```python
from build123d import *

# Parameters (mm, degrees)
BOSS_EXTRUDE1_DEPTH      = 4.9
BOSS_EXTRUDE1_DEPTH_BACK = 4.9


with BuildPart() as part:
    # Sketch1 → Boss-Extrude1 (new, two sides: drawn at the far end of the back side and taken through both)
    with BuildSketch(Plane(origin=(0, 0, 0), x_dir=(1, 0, 0), z_dir=(0, 1, 0)).offset(-BOSS_EXTRUDE1_DEPTH_BACK)):
        with BuildLine():
            Line((14.139704236, -107.57296828), (14.139704236, -55))
            Line((14.139704236, -55), (11.139704236, -55))
            Line((11.139704236, -55), (11.139704236, -107.57296828))
            ThreePointArc((11.139704236, -107.57296828), (11.954116062, -129.773650702), (14.392973543, -151.854989901))
            Line((14.392973543, -151.854989901), (34.78314741, -289.876871715))
            ThreePointArc((34.78314741, -289.876871715), (36.798345533, -293.542093696), (40.718726235, -295))
            Line((40.718726235, -295), (62.036020432, -295))
            ThreePointArc((62.036020432, -295), (63.863676368, -294.379006889), (64.934691141, -292.773115853))
            Line((64.934691141, -292.773115853), (69.645825561, -275.109492351))
            ThreePointArc((69.645825561, -275.109492351), (69.730627927, -274.02191122), (69.420940845, -272.975910231))
            Line((69.420940845, -272.975910231), (67.998466185, -270.180256335))
            Line((67.998466185, -270.180256335), (67.934740393, -270.07233274))
            Line((67.934740393, -270.07233274), (65.932760352, -266.681854911))
            ThreePointArc((65.932760352, -266.681854911), (65.317615772, -266.221021537), (64.557173026, -266.332811892))
            Line((64.557173026, -266.332811892), (63.276988126, -267.100922833))
            ThreePointArc((63.276988126, -267.100922833), (63.049164753, -267.408401483), (63.10548954, -267.786917173))
            Line((63.10548954, -267.786917173), (65.42072044, -271.645635339))
            Line((65.42072044, -271.645635339), (65.805438483, -272.286832078))
            ThreePointArc((65.805438483, -272.286832078), (65.89276832, -272.442724972), (65.970662013, -272.603540604))
            Line((65.970662013, -272.603540604), (66.311869933, -273.364986559))
            ThreePointArc((66.311869933, -273.364986559), (66.564497004, -274.351078344), (66.472838335, -275.364881152))
            Line((66.472838335, -275.364881152), (62.629961452, -289.773115853))
            ThreePointArc((62.629961452, -289.773115853), (61.558946679, -291.379006889), (59.731290743, -292))
            Line((59.731290743, -292), (43.308092042, -292))
            ThreePointArc((43.308092042, -292), (39.387711339, -290.542093696), (37.372513216, -286.876871715))
            Line((37.372513216, -286.876871715), (17.360762956, -151.416554044))
            ThreePointArc((17.360762956, -151.416554044), (14.946052579, -129.553841965), (14.139704236, -107.57296828))
        make_face()
    extrude(amount=BOSS_EXTRUDE1_DEPTH + BOSS_EXTRUDE1_DEPTH_BACK)


solid = part.part
```
Design review of the part built by this model. Coordinates are the model's own, in mm. A direction names the side the tool comes from. Give positions to 0.01 mm unless a question says otherwise; leave off trailing zeros. Loops run counter-clockwise (first coordinate to the right, second up) from the corner with the lowest first, then second, coordinate; pieces in that order, holes last. Notation, with made-up numbers: M -7.5,20 L 24.5,20 A10 ccw 24.5,29 Z; hole C -32.5,16 d7. An arc over 180 degrees is marked long. Return JSON: item names as keys, results as strings. Group by question number.
Item 1: We need section B-B (x = 56). Give the boundary of the cut face in (y, z), and give its area (3 significant figures).
Item 2: For probe 1 along Z at (x, y) = (56.5, 0.5); probe 2 along X at (y, z) = (2, 71); probe 3 along X at (y, z) = (3, 156), list the stretches that pass through material, from the lowest coordinate up.
Item 3: Insertion check: pin 1 Ø2 at (y, z) = (-1.5, 105) entering from +X; pin 2 Ø5 at (y, z) = (0.5, 166) entering from -X; pin 3 Ø2 at (x, y) = (39, -0.5) entering from +Z. Each pin has a flat end and moves straight along its axis. Give the tip position at first contact, or say it passes through.
Item 4: Tool access review of faces 5 (the flat face through (14.14, 0, 82)), 6 (the flat face through (64.578, -0.069, 282.468)), 7 (the flat face through (67.26, -0.07, 284.06)): name each direction out of +Z, -Z, +X, -X, +Y, -Y from which nothing blocks a thin tool from reaching the whole face with its end or side.
Item 5: We need section C-C (z = 264). Give the boundary of the cut face in (x, y), and give its area (3 significant figures).
Item 6: We need section A-A (y = -1.75). Give the boundary of the cut face in (x, z), and give its area (3 significant figures).
Item 7: Mouldability with a two-part tool opening along X and no side actions: class faces 1 (the flat face through (24.445, -0.069, 219.9)), 2 (the flat face through (52, 0, 292)), 3 (the cylindrical face through (39.43, -0.07, 290.58)), 4 (the cylindrical face through (14.97, -0.07, 129.86)) as released by +X, released by -X, zero draft, split by the parting line, or undercut.
Output:
{
 "1": {"outline": "M -4.9,292 L 4.9,292 L 4.9,295 L -4.9,295 Z", "area": "29.4 mm^2"},
 "2": {"probe 1": "z = 292 to 295", "probe 2": "x = 11.14 to 14.14", "probe 3": "x = 15.01 to 18.04"},
 "3": {"pin 1": "stops at x = 14.14", "pin 2": "stops at x = 16.11", "pin 3": "stops at z = 294.96"},
 "4": {"face 5": "-Z, +X, +Y, -Y", "face 6": "+Y, -Y", "face 7": "+Z, +X, +Y, -Y"},
 "5": {"outline": "M 30.96,-4.9 L 33.99,-4.9 L 33.99,4.9 L 30.96,4.9 Z", "area": "29.7 mm^2"},
 "6": {"outline": "M 11.14,55 L 14.14,55 L 14.14,107.57 A300 cw 17.36,151.42 L 37.37,286.88 A6 cw 43.31,292 L 59.73,292 A3 cw 62.63,289.77 L 66.47,275.36 A3 cw 66.31,273.36 L 65.97,272.6 A3 cw 65.81,272.29 L 63.11,267.79 A0.5 ccw 63.28,267.1 L 64.56,266.33 A1 ccw 65.93,266.68 L 68,270.18 L 69.42,272.98 A3 ccw 69.65,275.11 L 64.93,292.77 A3 ccw 62.04,295 L 40.72,295 A6 ccw 34.78,289.88 L 14.39,151.85 A303 ccw 11.14,107.57 Z", "area": "885 mm^2"},
 "7": {"face 1": "released by -X", "face 2": "undercut", "face 3": "undercut", "face 4": "released by +X"}
}
